Verification items for the finished model (mm, model axes). A direction names the side the tool comes from. Coordinates: 2 decimals unless noted, no trailing zeros. Loops run counter-clockwise (first coordinate to the right, second up) from the corner with the lowest first, then second, coordinate; pieces in that order, holes last. Notation, with made-up numbers: (76.25, -32) - (135.25, -32) arc R14 ccw to (135.25, -14) - close; hole circle Ø9 at (-20, 76.5). An arc over 180 degrees is marked (long way). One line per item, written item: value. Start each with the question number.
(1) Thickness scan on probe 1 along Y at (x, z) = (-35, 0.3); probe 2 along Z at (x, y) = (20.5, 19.5); probe 3 along X at (y, z) = (-26, 0.15). Record the ranges inside material, lowest first. Write a range as [from, to].
(2) Gauge pin test, flat ends, axial feed: P1, Ø1.5, axis at x = 35, y = 25, coming from the -Z side; P2, Ø8, axis at x = 24.5, y = 0, coming from the +Z side. Record the tip position at first contact, or that the pin passes through.
(3) Draft check along Y on faces 1 (the face through (0, 0, 0.5)), 2 (the face through (1, 0, 0)), 3 (the face through (-38.57, 28.5, 0.25)). Enter one of: +Y half, -Y half, draft (parallel to the pull), parting line (faces both ways), or undercut.
(4) Set-up check for faces 4 (the face through (0, 27, 0.5)), 5 (the face through (38.5, 28.57, 0.25)): record each of +Z, -Z, +X, -X, +Y, -Y from which the full face is reachable in a straight line by a thin tool's end or side.
(5) Section check A-A (y = -0.5). Record the boundary of the cut face in (x, z), plus the area to 3 significant figures.
(6) Section check B-B (x = -20.5). Record the boundary of the cut face in (y, z).
```python
from build123d import *

# Parameters (mm, degrees)
SKETCH_1_R      = 1.25
EXTRUDE_1_DEPTH = 0.5
EXTRUDE_5_DEPTH = 0.1


with BuildPart() as part:
    # 草图1 → 凸台-拉伸1 (new body)
    with BuildSketch(Plane.XY):
        with BuildLine():
            Line((-35, 30), (35, 30))
            ThreePointArc((35, 30), (38.535533906, 28.535533906), (40, 25))
            Line((40, 25), (40, -25))
            ThreePointArc((40, -25), (38.535533906, -28.535533906), (35, -30))
            Line((35, -30), (-35, -30))
            ThreePointArc((-35, -30), (-38.535533906, -28.535533906), (-40, -25))
            Line((-40, -25), (-40, 25))
            ThreePointArc((-40, 25), (-38.535533906, 28.535533906), (-35, 30))
        make_face()
        with Locations((35, 25)):
            Circle(SKETCH_1_R, mode=Mode.SUBTRACT)
        with Locations((-35, 25)):
            Circle(SKETCH_1_R, mode=Mode.SUBTRACT)
        with Locations((-35, -25)):
            Circle(SKETCH_1_R, mode=Mode.SUBTRACT)
        with Locations((35, -25)):
            Circle(SKETCH_1_R, mode=Mode.SUBTRACT)
    extrude(amount=EXTRUDE_1_DEPTH)

    # 草图4 → 凸台-拉伸5 (add)
    with BuildSketch(Plane.XY.offset(0.5)):
        with BuildLine():
            Line((-28.67544468, 25.1), (28.67544468, 25.1))
            ThreePointArc((28.67544468, 25.1), (29.667722556, 24.755143265), (30.232258297, 23.869230769))
            ThreePointArc((30.232258297, 23.869230769), (31.535176772, 21.535176772), (33.869230769, 20.232258297))
            ThreePointArc((33.869230769, 20.232258297), (34.755143265, 19.667722556), (35.1, 18.67544468))
            Line((35.1, 18.67544468), (35.1, -18.67544468))
            ThreePointArc((35.1, -18.67544468), (34.755143265, -19.667722556), (33.869230769, -20.232258297))
            ThreePointArc((33.869230769, -20.232258297), (31.535176772, -21.535176772), (30.232258297, -23.869230769))
            ThreePointArc((30.232258297, -23.869230769), (29.667722556, -24.755143265), (28.67544468, -25.1))
            Line((28.67544468, -25.1), (-28.67544468, -25.1))
            ThreePointArc((-28.67544468, -25.1), (-29.667722556, -24.755143265), (-30.232258297, -23.869230769))
            ThreePointArc((-30.232258297, -23.869230769), (-31.535176772, -21.535176772), (-33.869230769, -20.232258297))
            ThreePointArc((-33.869230769, -20.232258297), (-34.755143265, -19.667722556), (-35.1, -18.67544468))
            Line((-35.1, -18.67544468), (-35.1, 18.67544468))
            ThreePointArc((-35.1, 18.67544468), (-34.755143265, 19.667722556), (-33.869230769, 20.232258297))
            ThreePointArc((-33.869230769, 20.232258297), (-31.535176772, 21.535176772), (-30.232258297, 23.869230769))
            ThreePointArc((-30.232258297, 23.869230769), (-29.667722556, 24.755143265), (-28.67544468, 25.1))
        make_face()
        with BuildLine():
            Line((-28.67544468, 25), (28.67544468, 25))
            ThreePointArc((28.67544468, 25), (29.605705189, 24.676696811), (30.134957446, 23.846153846))
            ThreePointArc((30.134957446, 23.846153846), (31.464466094, 21.464466094), (33.846153846, 20.134957446))
            ThreePointArc((33.846153846, 20.134957446), (34.676696811, 19.605705189), (35, 18.67544468))
            Line((35, 18.67544468), (35, -18.67544468))
            ThreePointArc((35, -18.67544468), (34.676696811, -19.605705189), (33.846153846, -20.134957446))
            ThreePointArc((33.846153846, -20.134957446), (31.464466094, -21.464466094), (30.134957446, -23.846153846))
            ThreePointArc((30.134957446, -23.846153846), (29.605705189, -24.676696811), (28.67544468, -25))
            Line((28.67544468, -25), (-28.67544468, -25))
            ThreePointArc((-28.67544468, -25), (-29.605705189, -24.676696811), (-30.134957446, -23.846153846))
            ThreePointArc((-30.134957446, -23.846153846), (-31.464466094, -21.464466094), (-33.846153846, -20.134957446))
            ThreePointArc((-33.846153846, -20.134957446), (-34.676696811, -19.605705189), (-35, -18.67544468))
            Line((-35, -18.67544468), (-35, 18.67544468))
            ThreePointArc((-35, 18.67544468), (-34.676696811, 19.605705189), (-33.846153846, 20.134957446))
            ThreePointArc((-33.846153846, 20.134957446), (-31.464466094, 21.464466094), (-30.134957446, 23.846153846))
            ThreePointArc((-30.134957446, 23.846153846), (-29.605705189, 24.676696811), (-28.67544468, 25))
        make_face(mode=Mode.SUBTRACT)
    extrude(amount=EXTRUDE_5_DEPTH)


solid = part.part
```
Responses:
1. probe 1: y = [-30, -26.25], [-23.75, 23.75], [26.25, 30]
1. probe 2: z = [0, 0.5]
1. probe 3: x = [-39.9, -35.75], [-34.25, 34.25], [35.75, 39.9]
2. P1: passes through
2. P2: stops at z = 0.5
3. face 1: undercut
3. face 2: draft
3. face 3: +Y half
4. face 4: +Z
4. face 5: +Z, -Z, +X, +Y
5. outline: (-40, 0) - (40, 0) - (40, 0.5) - (35.1, 0.5) - (35.1, 0.6) - (35, 0.6) - (35, 0.5) - (-35, 0.5) - (-35, 0.6) - (-35.1, 0.6) - (-35.1, 0.5) - (-40, 0.5) - close
5. area: 40.0 mm²
6. outline: (-30, 0) - (30, 0) - (30, 0.5) - (25.1, 0.5) - (25.1, 0.6) - (25, 0.6) - (25, 0.5) - (-25, 0.5) - (-25, 0.6) - (-25.1, 0.6) - (-25.1, 0.5) - (-30, 0.5) - close
